Geometry check sheet. Reference: the model listing, model coordinates, mm. Coordinates: 2 decimals unless noted, no trailing zeros. Loops run counter-clockwise (first coordinate to the right, second up) from the corner with the lowest first, then second, coordinate; pieces in that order, holes last.
Autodesk Inventor part; units mm, degrees
ref_plane "YZ Plane" through (0, 0, 0) normal (1, 0, 0) x (0, 1, 0)
ref_plane "XZ Plane" through (0, 0, 0) normal (0, 1, 0) x (-1, 0, 0)
ref_plane "XY Plane" through (0, 0, 0) normal (0, 0, 1) x (1, 0, 0)
sketch "Sketch1" plane through (0, 0, 0) normal (0, 1, 0) x (-1, 0, 0)
  circle A0 centre (0, 50) radius 5
  circle A1 centre (0, 50) radius 10
  line L0 (-9.5533, 47.0447) -> (5, 0)
  line L1 (5, 0) -> (69.1187, 0)
  line L2 (69.1187, 6) -> (69.1187, 0)
  line L3 (69.1187, 6) -> (6.3595, 57.7173)
  point P0 (0, 0)
  dimension "d0" = 10
  dimension "d1" = 50
  dimension "d2" = 20
extrude "Extrusion1" add sketch "Sketch1" along normal mid plane 6
properties part number "Soporte resorte freno"
(1) Sectioned sample at B-B on z = 51. Record the cut outline in (x, y).
Findings:
outline: (-14.51, -3) - (-4.9, -3) - (-4.9, 3) - (-14.51, 3) - close; (4.9, -3) - (9.95, -3) - (9.95, 3) - (4.9, 3) - close
(2) Draft check along Z on faces 1 (the cylindrical face through (0.651, -0.042, 45.043)), 2 (the flat face through (2.38, -0.04, 23.85)), 3 (the cylindrical face through (6, 0, 58)), 4 (the flat face through (-20, -3, 24)). Enter one of: +Z half, -Z half, draft (parallel to the pull), parting line (faces both ways), or undercut.
Findings:
face 1: undercut
face 2: -Z half
face 3: parting line
face 4: draft
(3) Gauge pin test, flat ends, axial feed: pin 1 Ø1 at (x, y) = (-2, -0.5) entering from +Z; pin 2 Ø3 at (y, z) = (0.5, 20) entering from +X. Record the tip position at first contact, or that the pin passes through.
Findings:
pin 1: stops at z = 59.89
pin 2: stops at x = 1.65
(4) Sectioned sample at C-C on y = -1.2. Record the cut outline in (x, z).
Findings:
outline: (-69.12, 0) - (-5, 0) - (9.55, 47.04) arc R10 ccw to (-6.36, 57.72) - (-69.12, 6) - close; hole circle Ø10 at (0, 50)
(5) Sectioned sample at D-D on x = -47.5. Record the cut outline in (y, z), and give its area (3 significant figures).
Findings:
outline: (-3, 0) - (3, 0) - (3, 23.82) - (-3, 23.82) - close
area: 143 mm2
(6) Scan lines: L1, parallel to Z at x = -16.5, y = 2.2; L2, parallel to X at y = 2.65, z = 40.5; L3, parallel to Z at x = -9.5, y = -0.9. Record each from-to range of solid material in increasing order.
Findings:
L1: z = 0 to 49.36
L2: x = -27.25 to 7.53
L3: z = 0 to 55.13
(7) Sectioned sample at A-A on x = 0. Record the cut outline in (y, z), and give its area (3 significant figures).
Findings:
outline: (-3, 16.16) - (3, 16.16) - (3, 45) - (-3, 45) - close; (-3, 55) - (3, 55) - (3, 60) - (-3, 60) - close
area: 203 mm2
